from build123d import *

# Parameters (mm, degrees)
F1_DEPTH = 7.7


with BuildPart() as f1:
    # F0 (on Front) → F1 (new body)
    with BuildSketch(Plane.XZ):
        Polygon((-30.109993, 13.426532), (-36.756793, 13.426532), (-31.572289, -1.861103), (-21.73503, -13.16066), (-11.897769, -13.16066), (-22.266773, 0), align=None)
        Polygon((-31.572289, -1.861103), (-36.756793, 13.426532), (-36.756793, -4.963943), (-21.73503, -13.16066), align=None)
        Polygon((-11.897769, -13.16066), (-21.73503, -13.16066), (-15.544919, -15.920161), (-5.281532, -20.495497), (6.542794, -20.495497), align=None)
        Polygon((-15.544919, -15.920161), (-21.73503, -13.16066), (-24.515769, -20.495497), (-21.73503, -20.495497), align=None)
        Polygon((-5.281532, -20.495497), (-15.544919, -15.920161), (-21.73503, -20.495497), align=None)
    extrude(amount=F1_DEPTH)


solid = f1.part
For this review, take the finished solid that the model builds, in its own axes (mm). A direction names the side the tool comes from. Give positions to 0.01 mm unless a question says otherwise; leave off trailing zeros. Loops run counter-clockwise (first coordinate to the right, second up) from the corner with the lowest first, then second, coordinate; pieces in that order, holes last. Notation, with made-up numbers: (66.5, 38) -> (74.5, 38) arc R20 ccw to (74.5, 73) -> close; hole circle Ø9 at (42, 27). An arc over 180 degrees is marked (long way). One line per question, with ' | ' between items.
1) We need section D-D (x = 2.5). Write out the cut boundary in (y, z), plus the area to 3 significant figures.
Resolved:
outline: (-7.7, -20.5) -> (0, -20.5) -> (0, -18.89) -> (-7.7, -18.89) -> close | area: 12.4 mm2
2) We need section A-A (y = -6). Write out the cut boundary in (x, z), plus the area to 3 significant figures.
Resolved:
outline: (-36.76, -4.96) -> (-21.74, -13.16) -> (-24.52, -20.5) -> (6.54, -20.5) -> (-11.9, -13.16) -> (-22.27, 0) -> (-30.11, 13.43) -> (-36.76, 13.43) -> close | area: 489 mm2
3) The part is to be moulded in two halves that separate along Z. For faces 1 (the flat face through (-23.106, -3.796, -16.777)), 2 (the flat face through (-23, -7.7, -7)), 3 (the flat face through (-9, -4, -20.495)), 4 (the flat face through (-26.133, -3.796, 6.619)), say which applies: +Z half, -Z half, draft (parallel to the pull), parting line (faces both ways), or undercut.
Resolved:
face 1: undercut | face 2: draft | face 3: -Z half | face 4: +Z half
4) For faces 5 (the flat face through (-2.5, -3.8, -16.9)), 6 (the flat face through (-29.351, -3.796, -9.005)), list the 3-axis set-ups (+Z, -Z, +X, -X, +Y, -Y) from which the entire face can be reached by the end or side of a thin tool; tool diameter is ignored.
Resolved:
face 5: +Z, +X, +Y, -Y | face 6: -X, +Y, -Y
5) To check wall thickness, follow probe 1 along X at (y, z) = (-0.75, -9); probe 2 along X at (y, z) = (-3.75, 6.5); probe 3 along Z at (x, y) = (-25.5, -6.5). State the ranges of each line that lie inside material, in increasing order.
Resolved:
probe 1: x = -29.36 to -15.18 | probe 2: x = -36.76 to -26.06 | probe 3: z = -11.11 to 5.53
6) Insertion check: pin 1 Ø2 at (y, z) = (-2.5, -10) entering from +X; pin 2 Ø1 at (y, z) = (-5, -10) entering from -X. Each pin has a flat end and moves straight along its axis. Give the tip position at first contact, or say it passes through.
Resolved:
pin 1: stops at x = -13.6 | pin 2: stops at x = -28.44
7) We need section B-B (x = -23.5). Write out the cut boundary in (y, z).
Resolved:
outline: (-7.7, -20.5) -> (0, -20.5) -> (0, -17.82) -> (-7.7, -17.82) -> close; (-7.7, -12.2) -> (0, -12.2) -> (0, 2.11) -> (-7.7, 2.11) -> close
8) We need section C-C (z = -3.5). Write out the cut boundary in (x, y), plus the area to 3 significant figures.
Resolved:
outline: (-36.76, -7.7) -> (-19.51, -7.7) -> (-19.51, 0) -> (-36.76, 0) -> close | area: 133 mm2
